```python
from build123d import *

# Parameters (mm, degrees)
F0_R     = 63.5
F0_R_2   = 9.525
F0_R_3   = 31.75
F0_R_4   = 19.05
F1_DEPTH = 19.05
F2_DEPTH = 57.15
F3_DEPTH = 31.75
F4_DEPTH = 19.05
F5_DEPTH = 25.4


# Not quite as in the source:
# - ends of sketch curves that miss each other by under 0.0002 mm in the source are joined


with BuildPart() as f1:
    # F0 (on Top) → F1 (new body)
    with BuildSketch(Plane.XY):
        with BuildLine():
            ThreePointArc((2.2517e-06, -76.2), (53.8815375225, -53.8815359303), (76.2, 0))
            ThreePointArc((76.2, 0), (53.8815360903, 53.8815373625), (-1.7992e-06, 76.2))
            ThreePointArc((-1.7992e-06, 76.2), (-76.2, -2.0255e-06), (2.2517e-06, -76.2))
        make_face()
        Circle(F0_R, mode=Mode.SUBTRACT)
        with BuildLine():
            ThreePointArc((-1.7992e-06, 76.2), (53.8815360903, 53.8815373625), (76.2, 0))
            ThreePointArc((76.2, 0), (53.8815375225, -53.8815359303), (2.2517e-06, -76.2))
            Line((2.2517e-06, -76.2), (88.9, -76.199992084))
            Line((88.9, -76.199992084), (88.9, -38.100007916))
            Line((88.9, -38.100007916), (88.9, 38.100007916))
            Line((88.9, 38.100007916), (88.9, 76.200007916))
            Line((88.9, 76.200007916), (-1.7992e-06, 76.2))
        make_face()
        with BuildLine():
            ThreePointArc((2.2517e-06, -76.2), (-76.2, -2.0255e-06), (-1.7992e-06, 76.2))
            Line((-1.7992e-06, 76.2), (-88.9, 76.199992084))
            Line((-88.9, 76.199992084), (-88.9, 38.100007916))
            Line((-88.9, 38.100007916), (-88.9, -38.100007916))
            Line((-88.9, -38.100007916), (-88.9, -76.200007916))
            Line((-88.9, -76.200007916), (2.2517e-06, -76.2))
        make_face()
        with BuildLine():
            Line((-88.9, 38.100007916), (-88.9, 76.199992084))
            Line((-88.9, 76.199992084), (-107.95, 76.200007916))
            ThreePointArc((-107.95, 76.200007916), (-121.4203841816, 70.6203920976), (-127, 57.150007916))
            ThreePointArc((-127, 57.150007916), (-121.4203841816, 43.6796237344), (-107.95, 38.100007916))
            Line((-107.95, 38.100007916), (-88.9, 38.100007916))
        make_face()
        with Locations((-107.95, 57.150007916)):
            Circle(F0_R_2, mode=Mode.SUBTRACT)
        with BuildLine():
            Line((107.95, 76.200007916), (88.9, 76.200007916))
            Line((88.9, 76.200007916), (88.9, 38.100007916))
            Line((88.9, 38.100007916), (107.95, 38.100007916))
            ThreePointArc((107.95, 38.100007916), (121.4203841816, 43.6796237344), (127, 57.150007916))
            ThreePointArc((127, 57.150007916), (121.4203841816, 70.6203920976), (107.95, 76.200007916))
        make_face()
        with Locations((107.95, 57.150007916)):
            Circle(F0_R_2, mode=Mode.SUBTRACT)
        with BuildLine():
            Line((88.9, -38.100007916), (88.9, -76.199992084))
            Line((88.9, -76.199992084), (107.95, -76.200007916))
            ThreePointArc((107.95, -76.200007916), (121.4203841816, -70.6203920976), (127, -57.150007916))
            ThreePointArc((127, -57.150007916), (121.4203841816, -43.6796237344), (107.95, -38.100007916))
            Line((107.95, -38.100007916), (88.9, -38.100007916))
        make_face()
        with Locations((107.95, -57.150007916)):
            Circle(F0_R_2, mode=Mode.SUBTRACT)
        with BuildLine():
            Line((-107.95, -76.200007916), (-88.9, -76.200007916))
            Line((-88.9, -76.200007916), (-88.9, -38.100007916))
            Line((-88.9, -38.100007916), (-107.95, -38.100007916))
            ThreePointArc((-107.95, -38.100007916), (-121.4203841816, -43.6796237344), (-127, -57.150007916))
            ThreePointArc((-127, -57.150007916), (-121.4203841816, -70.6203920976), (-107.95, -76.200007916))
        make_face()
        with Locations((-107.95, -57.150007916)):
            Circle(F0_R_2, mode=Mode.SUBTRACT)
        Circle(F0_R)
        Circle(F0_R_3, mode=Mode.SUBTRACT)
        Circle(F0_R_3)
        Circle(F0_R_4, mode=Mode.SUBTRACT)
        Circle(F0_R_4)
        Circle(F0_R_2, mode=Mode.SUBTRACT)
        Circle(F0_R_2)
    extrude(amount=-F1_DEPTH)

    # F0 (on Top) → F2 (join)
    with BuildSketch(Plane.XY):
        with BuildLine():
            ThreePointArc((2.2517e-06, -76.2), (53.8815375225, -53.8815359303), (76.2, 0))
            ThreePointArc((76.2, 0), (53.8815360903, 53.8815373625), (-1.7992e-06, 76.2))
            ThreePointArc((-1.7992e-06, 76.2), (-76.2, -2.0255e-06), (2.2517e-06, -76.2))
        make_face()
        Circle(F0_R, mode=Mode.SUBTRACT)
    extrude(amount=F2_DEPTH)

    # F0 (on Top) → F3 (join)
    with BuildSketch(Plane.XY):
        Circle(F0_R_3)
        Circle(F0_R_4, mode=Mode.SUBTRACT)
    extrude(amount=F3_DEPTH)

    # F0 (on Top) → F4 (join)
    with BuildSketch(Plane.XY):
        Circle(F0_R_4)
        Circle(F0_R_2, mode=Mode.SUBTRACT)
    extrude(amount=F4_DEPTH)

    # F0 (on Top) → F5 (cut)
    with BuildSketch(Plane.XY):
        Circle(F0_R_2)
    extrude(amount=-F5_DEPTH, mode=Mode.SUBTRACT)


solid = f1.part
```
Part model, mm, in its own coordinate system. A direction names the side the tool comes from. Give positions to 0.01 mm unless a question says otherwise; leave off trailing zeros. Order: outer loops, then holes, each group sorted by start corner. A loop starts at its lowest first (then second) coordinate and runs counter-clockwise, first axis right, second up. Notation, with made-up numbers: M 48,48.25 L 92,48.25 A25 cw 92,81.25 Z; hole C 44,-30 d3. An arc over 180 degrees is marked long. Use a Markdown table: item, result. Add a question column.
(1) Saw through at A-A, the plane x = -92. Give the cut face in (y, z).
(2) Saw through at B-B, the plane y = 0. Give the cut face in (x, z) (3 decimals).
(3) Drop flat-ended pins along their axis: P1, Ø3, axis at y = -41.5, z = 26.5, coming from the +X side; P2, Ø21, axis at y = 8.5, z = -8, coming from the -X side; P3, Ø15, axis at y = -5, z = -13, coming from the +X side. Give the stop position or say it passes through.
(4) 3-axis set-ups, long thin cutter, end or side, ignore diameter. For faces 4 (the face through (98, 38.1, -9)), 5 (the face through (-99, 38.1, -9)), 6 (the face through (-15.12, -11.59, 25.31)), 7 (the face through (82, 0, 0)): which of +Z, -Z, +X, -X, +Y, -Y reach the whole face in a straight line?
(5) Saw through at C-C, the plane z = 24. Give the cut face in (x, y).
(6) Mould opens along Y. For faces 1 (the face through (-88.9, 1, -9)), 2 (the face through (35.162, -67.603, 28.175)), 3 (the face through (-29, 57, 57.15)) say: +Y half, -Y half, draft (parallel to the pull), parting line (faces both ways), or undercut.
(7) Probe line 1 along Y through (x, z) = (107, -10); line 2 along X through (y, z) = (1, 6); line 3 along Y through (x, z) = (0, 13.5) (3 decimals). List the from-to ranges inside material, lowest first. Write a range as [from, to].
(8) Saw through at D-D, the plane y = 61. Give the cut face in (x, z).
Answer key:
| question | item | result |
|---|---|---|
| 1 | outline | M -76.2,-19.05 L -38.1,-19.05 L -38.1,0 L -76.2,0 Z; M 38.1,-19.05 L 76.2,-19.05 L 76.2,0 L 38.1,0 Z |
| 2 | outline | M -88.9,-19.05 L -9.525,-19.05 L -9.525,19.05 L -19.05,19.05 L -19.05,31.75 L -31.75,31.75 L -31.75,0 L -63.5,0 L -63.5,57.15 L -76.2,57.15 L -76.2,0 L -88.9,0 Z; M 9.525,-19.05 L 88.9,-19.05 L 88.9,0 L 76.2,0 L 76.2,57.15 L 63.5,57.15 L 63.5,0 L 31.75,0 L 31.75,31.75 L 19.05,31.75 L 19.05,19.05 L 9.525,19.05 Z |
| 3 | P1 | x = 64.86 |
| 3 | P2 | x = -88.9 |
| 3 | P3 | x = 88.9 |
| 4 | face 4 | +Z, -Z, +X |
| 4 | face 5 | +Z, -Z, -X |
| 4 | face 6 | +Z |
| 4 | face 7 | +Z, +X |
| 5 | outline | C 0,0 d152.4; C 0,0 d63.5; hole C 0,0 d127; hole C 0,0 d38.1 |
| 6 | face 1 | undercut |
| 6 | face 2 | parting line |
| 6 | face 3 | draft |
| 7 | line 1 | [-76.2, -66.63], [-47.67, -38.1], [38.1, 47.67], [66.63, 76.2] |
| 7 | line 2 | [-76.19, -63.49], [-31.73, -9.47], [9.47, 31.73], [63.49, 76.19] |
| 7 | line 3 | [-76.2, -63.5], [-31.75, -9.525], [9.525, 31.75], [63.5, 76.2] |
| 8 | outline | M -126.61,-19.05 L -116.66,-19.05 L -116.66,0 L -126.61,0 Z; M -99.24,-19.05 L 99.24,-19.05 L 99.24,0 L 45.67,0 L 45.67,57.15 L 17.64,57.15 L 17.64,0 L -17.64,0 L -17.64,57.15 L -45.67,57.15 L -45.67,0 L -99.24,0 Z; M 116.66,-19.05 L 126.61,-19.05 L 126.61,0 L 116.66,0 Z |
